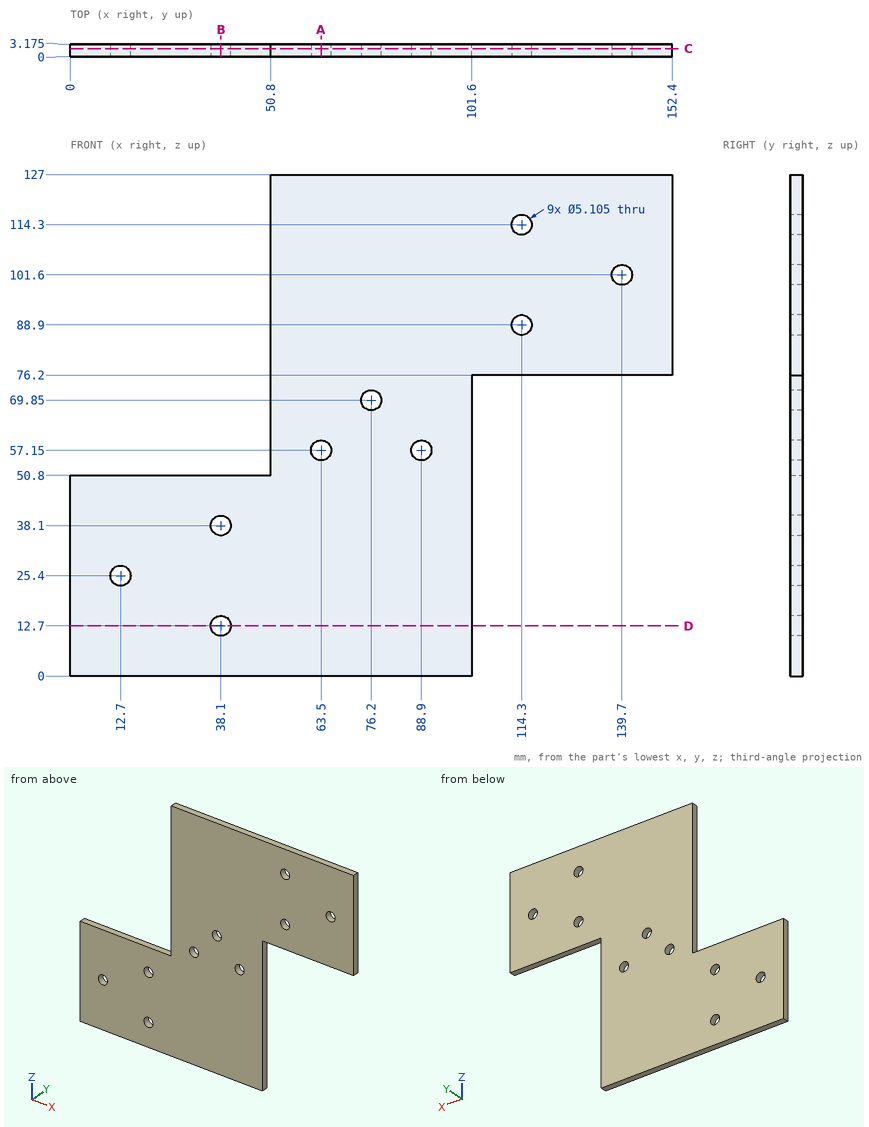
Source: three-view drawing plus pictorial views. Frame: mm from the lowest corner of the part. Coordinates: 2 decimals unless noted, no trailing zeros. Loops run counter-clockwise (first coordinate to the right, second up) from the corner with the lowest first, then second, coordinate; pieces in that order, holes last. Notation, with made-up numbers: (-14, 70) -> (-5, 70) arc R9 cw to (-5, 82) -> close; hole circle Ø8 at (88, 24.25). An arc over 180 degrees is marked (long way). Answer in a Markdown table with one row per item. Add a question column.
Q1. Section C-C on y = 2. Give the number of separate pieces and of enclosed holes in the cut face, and give its area (3 significant figures).
Q2. Ray query, line 1 along X through (y, z) = (1.2, 57.15); line 2 along Z through (x, y) = (38.1, 2.2); line 3 along X through (y, z) = (1.8, 69.85). Return the intervals inside material, ascending.
Q3. Contact query for a flat-ended pin moving along its axis: pin 1 Ø1.6 at (y, z) = (1.5, 80) entering from -X. Output: stop coordinate, or through.
Q4. Section A-A on x = 63.5. Return the cut outline in (y, z) (1 decimal).
Q5. Section D-D on z = 12.7. Return the cut outline in (x, y) (1 decimal).
Q6. Section B-B on x = 38.1. Return the cut outline in (y, z) (1 decimal).
Computed values:
| question | item | result |
|---|---|---|
| 1 | separate pieces | 1 |
| 1 | enclosed holes | 9 |
| 1 | area | 11,400 mm^2 |
| 2 | line 1 | x = 50.8 to 60.95, 66.05 to 86.35, 91.45 to 101.6 |
| 2 | line 2 | z = 0 to 10.15, 15.25 to 35.55, 40.65 to 50.8 |
| 2 | line 3 | x = 50.8 to 73.65, 78.75 to 101.6 |
| 3 | pin 1 | stops at x = 50.8 |
| 4 | outline | (0, 0) -> (3.2, 0) -> (3.2, 54.6) -> (0, 54.6) -> close; (0, 59.7) -> (3.2, 59.7) -> (3.2, 127) -> (0, 127) -> close |
| 5 | outline | (0, 0) -> (35.5, 0) -> (35.5, 3.2) -> (0, 3.2) -> close; (40.7, 0) -> (101.6, 0) -> (101.6, 3.2) -> (40.7, 3.2) -> close |
| 6 | outline | (0, 0) -> (3.2, 0) -> (3.2, 10.1) -> (0, 10.1) -> close; (0, 15.3) -> (3.2, 15.3) -> (3.2, 35.5) -> (0, 35.5) -> close; (0, 40.7) -> (3.2, 40.7) -> (3.2, 50.8) -> (0, 50.8) -> close |
